Could you check a few things on this drawing? It's one solid part, dimensions in mm from its lowest x, y, z. Give positions to 0.01 mm unless a question says otherwise; leave off trailing zeros. Loops run counter-clockwise (first coordinate to the right, second up) from the corner with the lowest first, then second, coordinate; pieces in that order, holes last. Notation, with made-up numbers: (1.25, 45) - (51.25, 45) arc R21 cw to (51.25, 54) - close; hole circle Ø2 at (-16, 17.25). An arc over 180 degrees is marked (long way). Put each result on its own line as item: value. Start each with the question number.
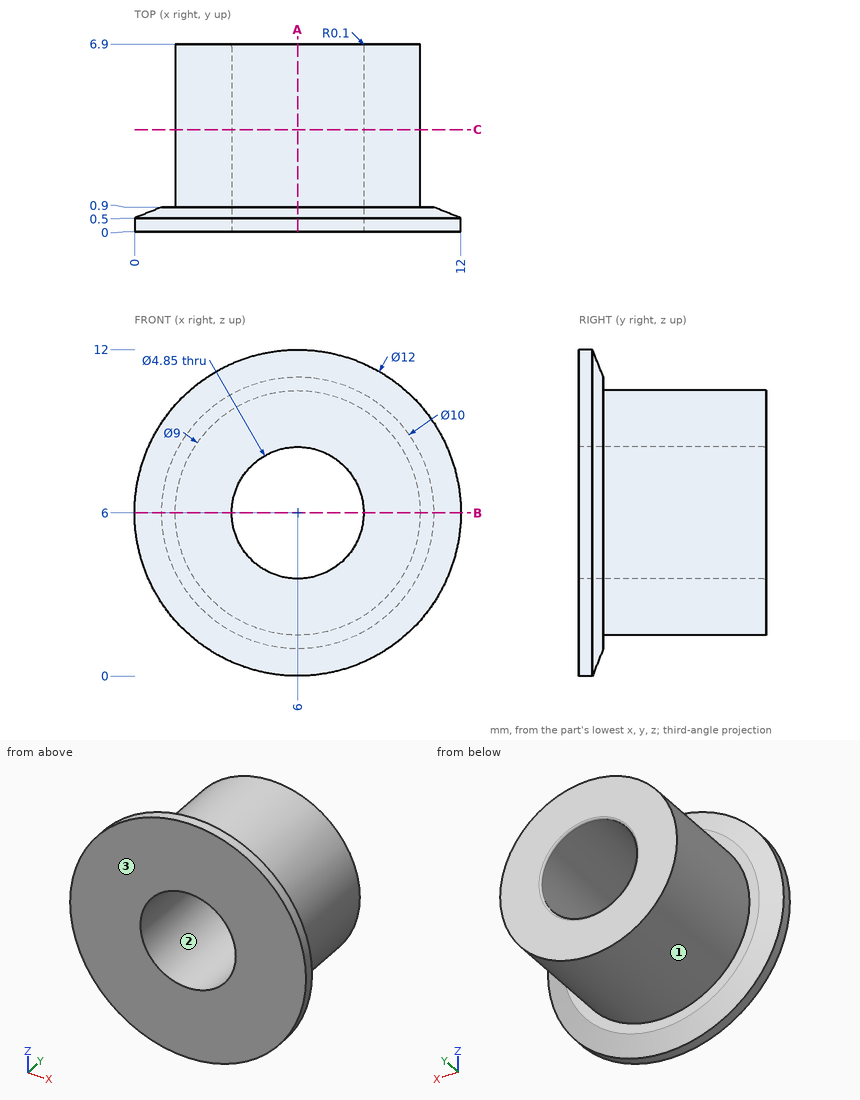
1) Suppose I cut it at C-C on y = 3.75. Please give me the cut outline in (x, z) (3 decimals).
2) Thinking about a two-plate mould opening in Z: for the marked faces 1, 2 and 3, which applies, pulls with the +Z half, pulls with the -Z half, needs draft (parallel to the pull), parting line crosses it, or undercut?
3) I'm going to push flat-ended pins straight in: P1, Ø4, axis at x = 8.5, y = 3.5, coming from the +Z side; P2, Ø2, axis at x = 9.5, y = 3, coming from the +Z side; P3, Ø1, axis at x = 2, y = 4.5, coming from the -Z side. Where does each tip first touch, or does it pass through?
4) Suppose I cut it at A-A on x = 6. Please give me the cut outline in (y, z) (3 decimals), plus the area to 3 significant figures.
5) I need wall thicknesses on line 1 (Z direction, x = 6, y = 5.25) (3 decimals); line 2 (Y direction, x = 7.25, z = 10.5). Which ranges of each line are inside material? Lowest first, please.
6) Suppose I cut it at B-B on z = 6. Please give me the cut outline in (x, y) (3 decimals), plus the area to 3 significant figures.
Ans:
1. outline: circle Ø9 at (6, 6); hole circle Ø4.85 at (6, 6)
2. face 1: parting line crosses it
2. face 2: undercut
2. face 3: needs draft
3. P1: stops at z = 10.47
3. P2: stops at z = 9.74
3. P3: stops at z = 3.17
4. outline: (0, 0) - (0.5, 0) - (0.9, 1) - (0.9, 1.5) - (6.9, 1.5) - (6.9, 3.475) arc R0.1 ccw to (6.8, 3.575) - (0, 3.575) - close; (0, 8.425) - (6.8, 8.425) arc R0.1 ccw to (6.9, 8.525) - (6.9, 10.5) - (0.9, 10.5) - (0.9, 11) - (0.5, 12) - (0, 12) - close
4. area: 30.9 mm²
5. line 1: z = 1.5 to 3.575, 8.425 to 10.5
5. line 2: y = 0 to 0.9
6. outline: (0, 0) - (3.575, 0) - (3.575, 6.8) arc R0.1 ccw to (3.475, 6.9) - (1.5, 6.9) - (1.5, 0.9) - (1, 0.9) - (0, 0.5) - close; (8.425, 0) - (12, 0) - (12, 0.5) - (11, 0.9) - (10.5, 0.9) - (10.5, 6.9) - (8.525, 6.9) arc R0.1 ccw to (8.425, 6.8) - close
6. area: 30.9 mm²
